The figure shows three views and two pictorial views of one solid part (mm, origin at its lowest corner). Answer the questions. Give positions to 0.01 mm unless a question says otherwise; leave off trailing zeros. Loops run counter-clockwise (first coordinate to the right, second up) from the corner with the lowest first, then second, coordinate; pieces in that order, holes last. Notation, with made-up numbers: (85.5, 21.5) - (133.5, 21.5) arc R29 ccw to (133.5, 49.5) - close; hole circle Ø2 at (5.25, -7). An arc over 180 degrees is marked (long way). One line per question, with ' | ' between items.
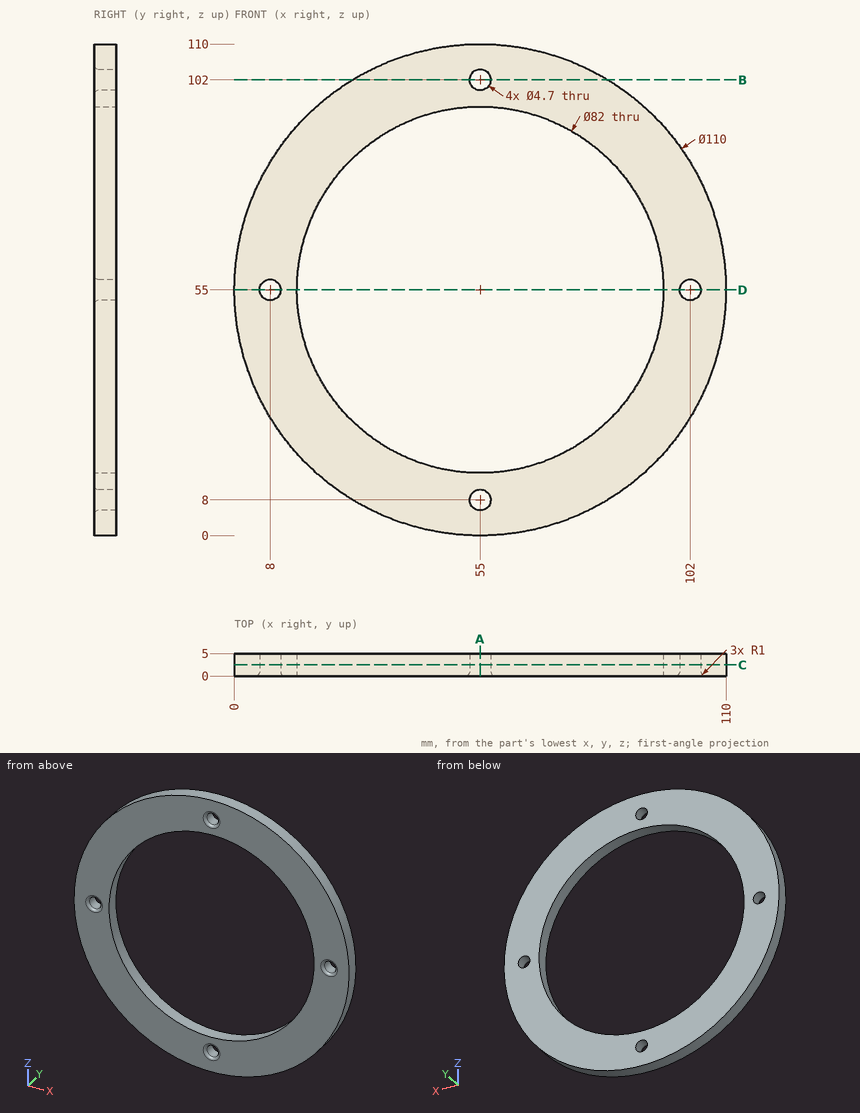
1. Flat-ended cylindrical pins translate along their axes: pin 1 (1.5 mm diameter, centred on y = 1, z = 93.5, fed in from +X); pin 2 (6 mm diameter, centred on x = 55, z = 102, fed in from -Y); pin 3 (3 mm diameter, centred on y = 1.5, z = 59.5, fed in from -X). Find the tip coordinate at first contact, or state that the pin passes through.
Evaluation:
pin 1: x = 95 | pin 2: y = 0.06 | pin 3: x = 0.08
2. Find section C-C on y = 2.5. Write down the section's boundary in (x, z).
Evaluation:
outline: circle Ø110 at (55, 55); hole circle Ø4.7 at (8, 55); hole circle Ø82 at (55, 55); hole circle Ø4.7 at (55, 8); hole circle Ø4.7 at (55, 102); hole circle Ø4.7 at (102, 55)
3. Find section A-A on x = 55. Write down the section's boundary in (y, z).
Evaluation:
outline: (0, 0) - (5, 0) - (5, 5.65) - (1, 5.65) arc R1 ccw to (0, 4.65) - close; (0, 11.35) arc R1 ccw to (1, 10.35) - (5, 10.35) - (5, 14) - (0, 14) - close; (0, 96) - (5, 96) - (5, 99.65) - (1, 99.65) arc R1 ccw to (0, 98.65) - close; (0, 105.35) arc R1 ccw to (1, 104.35) - (5, 104.35) - (5, 110) - (0, 110) - close
4. Find section B-B on z = 102. Write down the section's boundary in (x, y).
Evaluation:
outline: (26.43, 0) - (51.65, 0) arc R1 ccw to (52.65, 1) - (52.65, 5) - (26.43, 5) - close; (57.35, 1) arc R1 ccw to (58.35, 0) - (83.57, 0) - (83.57, 5) - (57.35, 5) - close
5. Consider L1, parallel to X at y = 2.15, z = 55; L2, parallel to X at y = 1, z = 18.5; L3, parallel to X at y = 1, z = 62.5. Determine where each line is inside the solid, lowest interval first.
Evaluation:
L1: 0 to 5.65, 10.35 to 14, 96 to 99.65, 104.35 to 110 | L2: 13.86 to 36.33, 73.67 to 96.14 | L3: 0.51 to 14.69, 95.31 to 109.49
6. Find section D-D on z = 55. Write down the section's boundary in (x, y).
Evaluation:
outline: (0, 0) - (4.65, 0) arc R1 ccw to (5.65, 1) - (5.65, 5) - (0, 5) - close; (10.35, 1) arc R1 ccw to (11.35, 0) - (14, 0) - (14, 5) - (10.35, 5) - close; (96, 0) - (98.65, 0) arc R1 ccw to (99.65, 1) - (99.65, 5) - (96, 5) - close; (104.35, 1) arc R1 ccw to (105.35, 0) - (110, 0) - (110, 5) - (104.35, 5) - close
